Here's how the part is built. I have some questions about the finished solid (model axes, mm). Face numbers are marked on the shaded views. A direction names the side the tool comes from. Give positions to 0.01 mm unless a question says otherwise; leave off trailing zeros. Loops run counter-clockwise (first coordinate to the right, second up) from the corner with the lowest first, then second, coordinate; pieces in that order, holes last.
Q1. For the marked faces 5, 6 and 7, which set-ups out of +Z, -Z, +X, -X, +Y, -Y let a thin tool reach every point of the face, with its end or its side?
Q2. Thinking about a two-plate mould opening in Y: for the marked faces 1, 2, 3 and 4, which applies, pulls with the +Y half, pulls with the -Y half, needs draft (parallel to the pull), parting line crosses it, or undercut?
Q3. Suppose I cut it at C-C (x = 1.8). List the corners of the cut face in (y, z) for me, and give its area (3 significant figures).
Q4. Suppose I cut it at B-B (y = 0). List the corners of the cut face in (x, z) for me.
Q5. I'm going to push a flat-ended pin straight in: P1, Ø0.6, axis at x = 1.5, z = -5, coming from the -Y side. Where does the tip first touch, or does it pass through?
Q6. I need wall thicknesses on probe 1 along Y at (x, z) = (1, 0); probe 2 along Y at (x, z) = (0.1, -4); probe 3 along Z at (x, y) = (0.2, 1.15). Which ranges of each line are inside material? Lowest first, please.
Q7. Suppose I cut it at D-D (y = -0.8). List the corners of the cut face in (x, z) for me, and give its area (3 significant figures).
Q8. Suppose I cut it at A-A (z = 0). List the corners of the cut face in (x, y) for me, and give its area (3 significant figures).
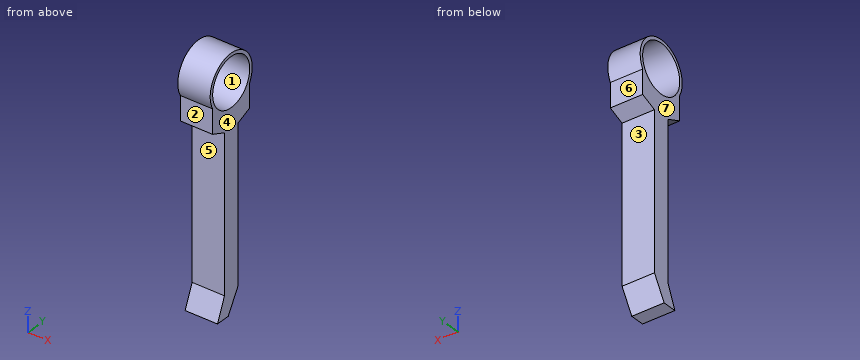
```python
from build123d import *

# Parameters (mm, degrees)
CROQUIS2_R              = 1.5
SALIENTE_EXTRUIR1_DEPTH = 2


with BuildPart() as part:
    # Croquis2 → Saliente-Extruir1 (new body)
    with BuildSketch(Plane(origin=(0, 0, 0), x_dir=(0, 0, -1), z_dir=(1, 0, 0))):
        with BuildLine():
            Line((2.289585189, 1.5), (0.8, 1.5))
            ThreePointArc((0.8, 1.5), (-1.7, 0), (0.8, -1.5))
            Line((0.8, -1.5), (2.289585189, -1.5))
            Line((2.289585189, -1.5), (2.688008385, -0.543556392))
            Line((2.688008385, -0.543556392), (12.241709619, -0.543556392))
            Line((12.241709619, -0.543556392), (13.6, -1.109375841))
            Line((13.6, -1.109375841), (13.6, -0.237921662))
            Line((13.6, -0.237921662), (12.241709619, 0.543556392))
            Line((12.241709619, 0.543556392), (2.688008385, 0.543556392))
            Line((2.688008385, 0.543556392), (2.289585189, 1.5))
        make_face()
        Circle(CROQUIS2_R, mode=Mode.SUBTRACT)
    extrude(amount=SALIENTE_EXTRUIR1_DEPTH)


solid = part.part
```
Solutions:
1. face 5: +X, -X, -Y
1. face 6: -Z, +X, -X, +Y
1. face 7: +Z, -Z, -X, +Y, -Y
2. face 1: undercut
2. face 2: pulls with the -Y half
2. face 3: pulls with the +Y half
2. face 4: needs draft
3. outline: (-1.5, -2.29) - (-0.54, -2.69) - (-0.54, -12.24) - (-1.11, -13.6) - (-0.24, -13.6) - (0.54, -12.24) - (0.54, -2.69) - (1.5, -2.29) - (1.5, -0.8) arc R1.7 ccw (long way) to (-1.5, -0.8) - close; hole circle Ø3 at (0, 0)
3. area: 17.1 mm2
4. outline: (0, -13.19) - (2, -13.19) - (2, -1.5) - (0, -1.5) - close; (0, 1.5) - (2, 1.5) - (2, 1.7) - (0, 1.7) - close
5. P1: stops at y = -0.54
6. probe 1: y = -1.7 to -1.5, 1.5 to 1.7
6. probe 2: y = -0.54 to 0.54
6. probe 3: z = -2.44 to -0.96, 0.96 to 1.25
7. outline: (0, -13.6) - (2, -13.6) - (2, -12.86) - (0, -12.86) - close; (0, -2.58) - (2, -2.58) - (2, -1.27) - (0, -1.27) - close; (0, 1.27) - (2, 1.27) - (2, 1.5) - (0, 1.5) - close
7. area: 4.57 mm2
8. outline: (0, -1.7) - (2, -1.7) - (2, -1.5) - (0, -1.5) - close; (0, 1.5) - (2, 1.5) - (2, 1.7) - (0, 1.7) - close
8. area: 0.800 mm2
